```python
from build123d import *

# Parameters (mm, degrees)
SKETCH1_W           = 34
SKETCH1_H           = 29
BOSS_EXTRUDE1_DEPTH = 4
SKETCH2_W           = 26
SKETCH2_H           = 23
CUT_EXTRUDE1_DEPTH  = 45.866468548
SKETCH3_W           = 32
SKETCH3_H           = 2
CUT_EXTRUDE2_DEPTH  = 28
BOSS_EXTRUDE2_DEPTH = 34
SKETCH5_R           = 1.75
CUT_EXTRUDE3_DEPTH  = 48.138094998
SKETCH6_W           = 14
SKETCH6_H           = 4
CUT_EXTRUDE4_DEPTH  = 5


with BuildPart() as part:
    # Sketch1 → Boss-Extrude1 (new body)
    with BuildSketch(Plane(origin=(0, 0, 0), x_dir=(1, 0, 0), z_dir=(0, 1, 0))):
        with Locations((17, 14.5)):
            Rectangle(SKETCH1_W, SKETCH1_H)
    extrude(amount=BOSS_EXTRUDE1_DEPTH)

    # Sketch2 → Cut-Extrude1 (cut, through all)
    with BuildSketch(Plane(origin=(0, 4, 0), x_dir=(1, 0, 0), z_dir=(0, 1, 0))):
        with Locations((17, 17.5)):
            Rectangle(SKETCH2_W, SKETCH2_H)
    extrude(amount=-CUT_EXTRUDE1_DEPTH, mode=Mode.SUBTRACT)

    # Sketch3 → Cut-Extrude2 (cut)
    with BuildSketch(Plane(origin=(0, 0, -29), x_dir=(-1, 0, 0), z_dir=(0, 0, -1))):
        with Locations((-17, 2)):
            Rectangle(SKETCH3_W, SKETCH3_H)
    extrude(amount=-CUT_EXTRUDE2_DEPTH, mode=Mode.SUBTRACT)

    # Sketch4 → Boss-Extrude2 (add)
    with BuildSketch(Plane.ZY):
        Polygon((0, 4), (3, 4), (3, -15), (0, -15), (0, 0), align=None)
    extrude(amount=-BOSS_EXTRUDE2_DEPTH)

    # Sketch5 → Cut-Extrude3 (cut, through all)
    with BuildSketch(Plane(origin=(0, 0, 0), x_dir=(-1, 0, 0), z_dir=(0, 0, -1))):
        with Locations(Location((-29.5, -10, 0), (0, 0, 90))):
            Circle(SKETCH5_R)
        with Locations(Location((-4.5, -10, 0), (0, 0, 90))):
            Circle(SKETCH5_R)
    extrude(amount=-CUT_EXTRUDE3_DEPTH, mode=Mode.SUBTRACT)

    # Sketch6 → Cut-Extrude4 (cut)
    with BuildSketch(Plane(origin=(0, 0, -6), x_dir=(-1, 0, 0), z_dir=(0, 0, -1))):
        with Locations((-17, 2)):
            Rectangle(SKETCH6_W, SKETCH6_H)
    extrude(amount=-CUT_EXTRUDE4_DEPTH, mode=Mode.SUBTRACT)


solid = part.part
```
For this review, take the finished solid that the model builds, in its own axes (mm). A direction names the side the tool comes from. Give positions to 0.01 mm unless a question says otherwise; leave off trailing zeros. Write each loop counter-clockwise with the first axis right and the second up, starting at its lowest first coordinate (ties: lowest second). Pieces come first, ordered by that corner, then holes.
Item 1: Machinability: for faces 1 (the face through (10, 0.5, -3.5)), 2 (the face through (17, -5, 3)), 3 (the face through (1, 2, -15)), which of the approach directions +Z, -Z, +X, -X, +Y, -Y give a long, thin tool a straight path to every point of the face, cutting with its end or side? Answer none if there is none.
Item 2: The part is to be moulded in two halves that separate along X. For faces 4 (the face through (33.3, 2, -29)), 5 (the face through (30, 0.5, -17.3)), 6 (the face through (34, 0.2, -9.4)), 7 (the face through (0, 0.2, -9.4)), say which applies: +X half, -X half, draft (parallel to the pull), parting line (faces both ways), or undercut.
Item 3: Insertion check: P1, Ø10, axis at x = 6, z = -10, coming from the -Y side; P2, Ø0.8, axis at x = 7.5, y = 3.5, coming from the -Z side. Each pin has a flat end and moves straight along its axis. Give the tip position at first contact, or say it passes through.
Item 4: Take a section at B-B (x = 29.5). Give the boundary of the cut face in (y, z).
Item 5: Take a section at A-A (z = -4). Give the boundary of the cut face in (x, y).
Item 6: Wall thickness on probe 1 along X at (y, z) = (-10, 1.3); probe 2 along Z at (x, y) = (10, -4.25); probe 3 along Y at (x, z) = (4, 1): over which ranges is each line inside the solid? List them lowest first.
Item 7: Take a section at D-D (x = 9.5). Give the boundary of the cut face in (y, z), and give its area (3 significant figures).
Item 8: Take a section at C-C (y = -10). Give the boundary of the cut face in (x, z), and give its area (3 significant figures).
Established:
1. face 1: -Z, +Y, -Y
1. face 2: +Z, +X, -X, +Y, -Y
1. face 3: -Z
2. face 4: draft
2. face 5: undercut
2. face 6: +X half
2. face 7: -X half
3. P1: stops at y = 0
3. P2: stops at z = -6
4. outline: (-15, 0) - (-11.75, 0) - (-11.75, 3) - (-15, 3) - close; (-8.25, 0) - (0, 0) - (0, -6) - (1, -6) - (1, -1) - (3, -1) - (3, -6) - (4, -6) - (4, 3) - (-8.25, 3) - close
5. outline: (0, 0) - (10, 0) - (10, 1) - (1, 1) - (1, 3) - (10, 3) - (10, 4) - (0, 4) - close; (24, 0) - (34, 0) - (34, 4) - (24, 4) - (24, 3) - (33, 3) - (33, 1) - (24, 1) - close
6. probe 1: x = 0 to 2.75, 6.25 to 27.75, 31.25 to 34
6. probe 2: z = 0 to 3
6. probe 3: y = -15 to -11.68, -8.32 to 4
7. outline: (-15, 0) - (0, 0) - (0, -6) - (1, -6) - (1, -1) - (3, -1) - (3, -6) - (4, -6) - (4, 3) - (-15, 3) - close
7. area: 71.0 mm2
8. outline: (0, 0) - (2.75, 0) - (2.75, 3) - (0, 3) - close; (6.25, 0) - (27.75, 0) - (27.75, 3) - (6.25, 3) - close; (31.25, 0) - (34, 0) - (34, 3) - (31.25, 3) - close
8. area: 81.0 mm2
